Could you check a few things on this model? Use its own coordinates, in mm. A direction names the side the tool comes from. Coordinates: 2 decimals unless noted, no trailing zeros. Loops run counter-clockwise (first coordinate to the right, second up) from the corner with the lowest first, then second, coordinate; pieces in that order, holes last. Notation, with made-up numbers: (-38, 81.25) - (-10, 81.25) arc R22 cw to (-10, 109.25) - close; hole circle Ø9 at (-6.75, 73.5). An arc over 180 degrees is marked (long way). One line per question, with ' | ' between items. Start each with the question number.
1. I want a section at A-A, the plane x = 104. Write out the boundary of the cut face in (y, z).
2. I want a section at D-D, the plane x = 50. Write out the boundary of the cut face in (y, z).
3. I want a section at C-C, the plane y = 16.25. Count the separate pieces of the cut face and the enclosed holes in it, then the cut area to 3 significant figures.
4. I'm going to push flat-ended pins straight in: P1, Ø5, axis at x = 81.5, y = 18, coming from the -Z side; P2, Ø1, axis at y = 16.5, z = -3.5, coming from the +X side. Where does each tip first touch, or does it pass through?
5. Please list where these lines run through material, in increasing order: L1, parallel to Y at x = 73.05, z = 0.7; L2, parallel to X at y = 2.25, z = -2.5; L3, parallel to Z at x = 104, y = 14. Write a range as [from, to].
6. I want a section at B-B, the plane x = 34.95. Write out the boundary of the cut face in (y, z), then the cut area to 3 significant figures.
7. Which directions (+Z, -Z, +X, -X, +Y, -Y) give clear straight access to the entire face, cutting with the end or side of a thin tool? Please do faces 1 (the flat face through (54, 0, 1)), 2 (the flat face through (46.5, 4, 1)), 3 (the flat face through (53, 13, 0)).
8. We'd pull the mould along Z, two halves only. Please class faces 4 (the cylindrical face through (104.584, 12.675, -5.957)), 5 (the flat face through (53, 13, 2)), 6 (the flat face through (54, 25, 1)), 7 (the cylindrical face through (2.25, 12.68, -2.08)): pulls with the +Z half, pulls with the -Z half, needs draft (parallel to the pull), parting line crosses it, or undercut.
Autodesk Inventor part; units mm, degrees
ref_plane "YZ Plane" through (0, 0, 0) normal (1, 0, 0) x (0, 1, 0)
ref_plane "XZ Plane" through (0, 0, 0) normal (0, 1, 0) x (-1, 0, 0)
ref_plane "XY Plane" through (0, 0, 0) normal (0, 0, 1) x (1, 0, 0)
sketch "Skizze1" plane through (0, 0, 0) normal (0, 0, 1) x (1, 0, 0)
  line L0 (0, 0) -> (108, 0)
  line L1 (108, 0) -> (108, 25)
  line L2 (108, 25) -> (0, 25)
  line L3 (0, 25) -> (0, 0)
  dimension "d5" = 108
  dimension "d6" = 25
extrude "Extrusion1" add sketch "Skizze1" along normal blind 2
sketch "Skizze3" plane through (0, 25, 0) normal (0, 1, 0) x (1, 0, 0)
  circle A0 centre (4, 2) radius 1.75
  circle A1 centre (104, 2) radius 1.75
  line L0 (4, 2) -> (104, 2) construction
  line L1 (0, 0) -> (108, 0) construction
  line L2 (54, 0) -> (54, 2) construction
  line L3 (0, 0) -> (8, 0)
  line L4 (108, 0) -> (100, 0)
  line L5 (0, 0) -> (0, 2)
  line L6 (8, 2) -> (8, 0)
  line L7 (100, 2) -> (100, 0)
  line L8 (108, 0) -> (108, 2)
  arc A2 (8, 2) -> (0, 2) centre (4, 2) ccw
  arc A3 (108, 2) -> (100, 2) centre (104, 2) ccw
  dimension "d2" = 100
  dimension "d3" = 3.5
  dimension "d4" = 2
extrude "Extrusion2" add sketch "Skizze3" against normal up to surface (25 mm away)
sketch "Skizze4" plane through (0, 0, 2) normal (0, 0, 1) x (1, 0, 0)
  line L0 (34.95, 5.261) -> (73.05, 5.261) construction
  line L1 (73.05, 5.261) -> (73.05, 19.739) construction
  line L2 (73.05, 19.739) -> (34.95, 19.739) construction
  line L3 (34.95, 19.739) -> (34.95, 5.261) construction
  line L4 (108, 25) -> (0, 25) construction
  line L5 (54, 25) -> (54, 0) construction
  line L6 (0, 0) -> (108, 0) construction
  line L7 (0, 25) -> (0, 0) construction
  line L8 (0, 12.5) -> (108, 12.5) construction
  line L9 (108, 0) -> (108, 25) construction
  circle A0 centre (73.05, 19.739) radius 1.5
  circle A1 centre (34.95, 5.261) radius 1.5
  circle A2 centre (34.95, 19.739) radius 1.5
  circle A3 centre (73.05, 5.261) radius 1.5
  point P0 (54, 19.739)
  point P1 (73.05, 12.5)
  dimension "d12" = 38.1
  dimension "d13" = 14.478
  dimension "d14" = 3
extrude "Extrusion3" cut sketch "Skizze4" against normal blind 8
sketch "Skizze5" plane through (0, 0, 2) normal (0, 0, 1) x (1, 0, 0)
  line L0 (44.09, 22.4949) -> (0.91, 22.4949) construction
  line L1 (0.91, 22.4949) -> (0.91, 2.5051) construction
  line L2 (0.91, 2.5051) -> (44.09, 2.5051) construction
  line L3 (44.09, 2.5051) -> (44.09, 22.4949) construction
  line L4 (108, 25) -> (0, 25) construction
  line L5 (54, 25) -> (54, 0) construction
  line L6 (0, 0) -> (108, 0) construction
  line L7 (108, 0) -> (108, 25) construction
  line L8 (108, 12.5) -> (0, 12.5) construction
  line L9 (0, 25) -> (0, 0) construction
  line L10 (46.5, 6.0051) -> (61.5, 6.0051)
  line L11 (61.5, 6.0051) -> (61.5, 2.0051)
  line L12 (61.5, 2.0051) -> (46.5, 2.0051)
  line L13 (46.5, 2.0051) -> (46.5, 6.0051)
  point P0 (0.91, 12.5)
  point P1 (54, 6.0051)
  dimension "d17" = 43.18
  dimension "d18" = 19.9898
  dimension "d19" = 15
  dimension "d20" = 4
  dimension "d27" = 0.5
extrude "Extrusion4" cut sketch "Skizze5" against normal up to next
fillet "Rundung1" radius 1 4 edges at (46.5, 6.0051, 1) (61.5, 6.0051, 1) (61.5, 2.0051, 1) (46.5, 2.0051, 1)
fillet "Rundung2" radius 4 2 edges at (8, 12.5, 0) (100, 12.5, 0)
fillet "Rundung3" radius 1 2 edges at (0, 12.5, 2) (108, 12.5, 2)
properties part number "US Halterung hinten leicht" material "ABS-Kunststoff"
Results are:
1) outline: (0, -6) - (25, -6) - (25, -3.75) - (0, -3.75) - close; (0, -0.25) - (25, -0.25) - (25, 2) - (0, 2) - close
2) outline: (0, 0) - (2.01, 0) - (2.01, 2) - (0, 2) - close; (6.01, 0) - (25, 0) - (25, 2) - (6.01, 2) - close
3) separate pieces: 1 | enclosed holes: 2 | area: 284 mm2
4) P1: stops at z = 0 | P2: stops at x = 107.87
5) L1: y = [0, 3.76], [6.76, 18.24], [21.24, 25] | L2: x = [0.03, 2.32], [5.68, 8.04], [99.96, 102.32], [105.68, 107.97] | L3: z = [-6, -3.75], [-0.25, 2]
6) outline: (0, 0) - (3.76, 0) - (3.76, 2) - (0, 2) - close; (6.76, 0) - (18.24, 0) - (18.24, 2) - (6.76, 2) - close; (21.24, 0) - (25, 0) - (25, 2) - (21.24, 2) - close | area: 38.0 mm2
7) face 1: +Z, -Z, +X, -X, -Y | face 2: +Z, -Z | face 3: -Z, +Y, -Y
8) face 4: pulls with the -Z half | face 5: pulls with the +Z half | face 6: needs draft | face 7: undercut
